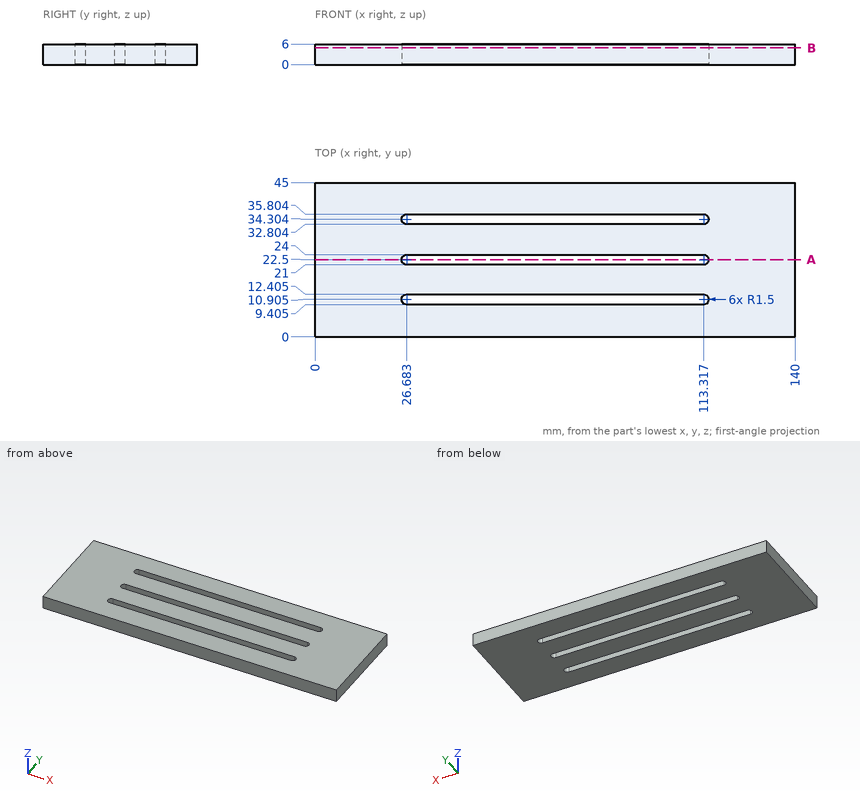
Can you work these out from the drawing? Everything is in mm from the part's minimum corner. Give positions to 0.01 mm unless a question says otherwise; leave off trailing zeros. Order: outer loops, then holes, each group sorted by start corner. A loop starts at its lowest first (then second) coordinate and runs counter-clockwise, first axis right, second up. Notation, with made-up numbers: M 64.5,-11 L 102.5,-11 A19 ccw 102.5,20 Z; hole C -5,15 d7. An arc over 180 degrees is marked long. Write item = value, one per line. Start each with the question number.
Q1. Suppose I cut it at A-A (y = 22.5). Write out the boundary of the cut face in (x, z), plus the area to 3 significant figures.
Q2. Will this pin go through, and if not, where does the flat tip stop? pin 1 Ø2 at (x, z) = (101.5, 3) entering from -Y.
Q3. I need wall thicknesses on probe 1 along Y at (x, z) = (90, 5.65) (1 decimal); probe 2 along X at (y, z) = (22.5, 2.15); probe 3 along X at (y, z) = (22, 4.1). Which ranges of each line are inside material? Lowest first, please. Write a range as [from, to].
Q4. Suppose I cut it at B-B (z = 4.9). Write out the boundary of the cut face in (x, y) (1 decimal), plus the area to 3 significant figures.
Check result:
q1.outline = M 0,0 L 25.18,0 L 25.18,6 L 0,6 Z; M 114.82,0 L 140,0 L 140,6 L 114.82,6 Z
q1.area = 302 mm2
q2.pin_1 = 0
q3.probe_1 = [0, 9.4], [12.4, 21], [24, 32.8], [35.8, 45]
q3.probe_2 = [0, 25.18], [114.82, 140]
q3.probe_3 = [0, 25.27], [114.73, 140]
q4.outline = M 0,0 L 140,0 L 140,45 L 0,45 Z; hole M 26.7,9.4 L 113.3,9.4 A1.5 ccw 113.3,12.4 L 26.7,12.4 A1.5 ccw Z; hole M 26.7,21 L 113.3,21 A1.5 ccw 113.3,24 L 26.7,24 A1.5 ccw Z; hole M 26.7,32.8 L 113.3,32.8 A1.5 ccw 113.3,35.8 L 26.7,35.8 A1.5 ccw Z
q4.area = 5,500 mm2
